The listing builds one solid part. Answer for the finished solid, in the listing's coordinates (mm). Face numbers are marked on the shaded views. Round coordinates to 2 decimals unless told otherwise and drop trailing zeros. Loops run counter-clockwise (first coordinate to the right, second up) from the corner with the lowest first, then second, coordinate; pieces in that order, holes last. Notation, with made-up numbers: M -17.75,18.25 L -7.75,18.25 A20 ccw -7.75,44.25 Z; hole C 36,59 d10. An arc over 180 degrees is marked long. Put each result on its own line as item: value. Start each with the question number.
(1) Straight lines are drawn through the part: line 1 (Z direction, x = 173.5, y = -11.25); line 2 (Z direction, x = 55.5, y = -12.5); line 3 (Z direction, x = 284.5, y = -13.75). For each, find the intervals that lie inside material, in ascending order.
(2) Section A-A, the plane x = 105 is taken. Determine the outline of the cut face in (y, z).
(3) Determine the mould class of the marked faces 1 and 2 for opening direction Z: released by +Z, released by -Z, zero draft, split by the parting line, or undercut.
(4) Section B-B, the plane z = 670 is taken. Determine the outline of the cut face in (x, y).
(5) Flat-ended cylindrical pins translate along their axes: P1, Ø8, axis at x = 130.5, z = 746.5, coming from the -Y side; P2, Ø1.5, axis at x = 344, y = -14, coming from the -Z side. Find the tip coordinate at first contact, or state that the pin passes through.
(6) Section C-C, the plane z = 704.5 is taken. Determine the outline of the cut face in (x, y), then the cut area to 3 significant figures.
```python
from build123d import *

# Parameters (mm, degrees)
F0_W      = 44.656470418
F0_H      = 33.8078811765
F1_DEPTH  = 16
F2_DEPTH  = 796
F3_DEPTH  = 196
F4_W      = 68.9578056335
F4_H      = 493.6993122101
F5_DEPTH  = 7
F6_DEPTH  = 9.7
F7_DEPTH  = 99.33
F8_DEPTH  = 99.33
F9_DEPTH  = 17.34
F10_DEPTH = 102.97
F11_W     = 35.2807044983
F11_H     = 492.0964837074
F12_DEPTH = 7
F13_DEPTH = 37.27
F14_DEPTH = 6.58
F15_DEPTH = 106.63
F16_DEPTH = 5.87
F17_DEPTH = 200
F18_DEPTH = 200
F19_DEPTH = 200
F20_DEPTH = 600
F21_DEPTH = 600
F22_DEPTH = 600
F23_R     = 3


with BuildPart() as f1:
    # F0 (on Front) → F1 (new body)
    with BuildSketch(Plane.XZ):
        with Locations((22.328235209, 16.9039405882)):
            Rectangle(F0_W, F0_H)
    extrude(amount=F1_DEPTH)

    # F2 (add): a face of the model
    f2_faces = [f1.faces().sort_by_distance(p)[0] for p in [
        (22.328235209, -8, 0),
    ]]
    extrude(f2_faces, amount=-F2_DEPTH)

    # F3 (add): a face of the model
    f3_faces = [f1.faces().sort_by_distance(p)[0] for p in [
        (0, -8, 398),
    ]]
    extrude(f3_faces, amount=-F3_DEPTH)

    # F4 (on face) → F5 (cut)
    with BuildSketch(Plane.XZ.offset(16)):
        with Locations((94.1769480705, 399.8196721077)):
            Rectangle(F4_W, F4_H)
    extrude(amount=-F5_DEPTH, mode=Mode.SUBTRACT)

    # F6 (cut): a face of the model
    f6_faces = [f1.faces().sort_by_distance(p)[0] for p in [
        (59.6980452538, -12.5, 399.8196721077),
    ]]
    extrude(f6_faces, amount=-F6_DEPTH, mode=Mode.SUBTRACT)

    # F7 (add): a face of the model
    f7_faces = [f1.faces().sort_by_distance(p)[0] for p in [
        (89.3269480705, -12.5, 646.6693282127),
    ]]
    extrude(f7_faces, amount=-F7_DEPTH)

    # F8 (cut): a face of the model
    f8_faces = [f1.faces().sort_by_distance(p)[0] for p in [
        (89.3269480705, -12.5, 646.6693282127),
    ]]
    extrude(f8_faces, amount=-F8_DEPTH, mode=Mode.SUBTRACT)

    # F9 (cut): a face of the model
    f9_faces = [f1.faces().sort_by_distance(p)[0] for p in [
        (128.6558508873, -12.5, 449.4846721077),
    ]]
    extrude(f9_faces, amount=-F9_DEPTH, mode=Mode.SUBTRACT)

    # F10 (cut): a face of the model
    f10_faces = [f1.faces().sort_by_distance(p)[0] for p in [
        (97.9969480705, -12.5, 152.9700160027),
    ]]
    extrude(f10_faces, amount=-F10_DEPTH, mode=Mode.SUBTRACT)

    # F11 (on face) → F12 (join)
    with BuildSketch(Plane.XZ.offset(9)):
        with Locations((91.7714834213, 432.6795041561)):
            Rectangle(F11_W, F11_H)
    extrude(amount=F12_DEPTH)

    # F13 (add): a face of the model
    f13_faces = [f1.faces().sort_by_distance(p)[0] for p in [
        (91.7714834213, -12.5, 678.7277460098),
    ]]
    extrude(f13_faces, amount=F13_DEPTH)

    # F14 (add): a face of the model
    f14_faces = [f1.faces().sort_by_distance(p)[0] for p in [
        (109.4118356705, -12.5, 451.3145041561),
    ]]
    extrude(f14_faces, amount=F14_DEPTH)

    # F15 (add): a face of the model
    f15_faces = [f1.faces().sort_by_distance(p)[0] for p in [
        (95.0614834213, -12.5, 186.6312623024),
    ]]
    extrude(f15_faces, amount=F15_DEPTH)

    # F16 (cut): a face of the model
    f16_faces = [f1.faces().sort_by_distance(p)[0] for p in [
        (74.1311311722, -12.5, 397.9995041561),
    ]]
    extrude(f16_faces, amount=-F16_DEPTH, mode=Mode.SUBTRACT)

    # F17 (add): a face of the model
    f17_faces = [f1.faces().sort_by_distance(p)[0] for p in [
        (196, -8, 398),
    ]]
    extrude(f17_faces, amount=F17_DEPTH)

    # F18 (cut): a face of the model
    f18_faces = [f1.faces().sort_by_distance(p)[0] for p in [
        (145.9958508873, -12.5, 397.9996721077),
    ]]
    extrude(f18_faces, amount=-F18_DEPTH, mode=Mode.SUBTRACT)

    # F19 (add): a face of the model
    f19_faces = [f1.faces().sort_by_distance(p)[0] for p in [
        (115.9918356705, -12.5, 397.9995041561),
    ]]
    extrude(f19_faces, amount=F19_DEPTH)

    # F20 (cut): a face of the model
    f20_faces = [f1.faces().sort_by_distance(p)[0] for p in [
        (197.9964834213, -12.5, 80.0012623024),
    ]]
    extrude(f20_faces, amount=-F20_DEPTH, mode=Mode.SUBTRACT)

    # F21 (add): a face of the model
    f21_faces = [f1.faces().sort_by_distance(p)[0] for p in [
        (197.9969480705, -12.5, 50.0000160027),
    ]]
    extrude(f21_faces, amount=F21_DEPTH)

    # F22 (cut): a face of the model
    f22_faces = [f1.faces().sort_by_distance(p)[0] for p in [
        (198, -8, 0),
    ]]
    extrude(f22_faces, amount=-F22_DEPTH, mode=Mode.SUBTRACT)

    # F23
    f23_edges = [f1.edges().sort_by_distance(p)[0] for p in [
        (0, -16, 698),
        (198, -16, 796),
        (396, -16, 698),
        (198, -16, 600),
        (197.996948, -16, 745.999328),
        (49.998045, -16, 697.999672),
        (345.995851, -16, 697.999672),
        (197.996948, -16, 650.000016),
        (197.996483, -16, 715.997746),
        (315.991836, -16, 697.999504),
        (197.996483, -16, 680.001262),
        (80.001131, -16, 697.999504),
    ]]
    fillet(f23_edges, radius=F23_R)


solid = f1.part
```
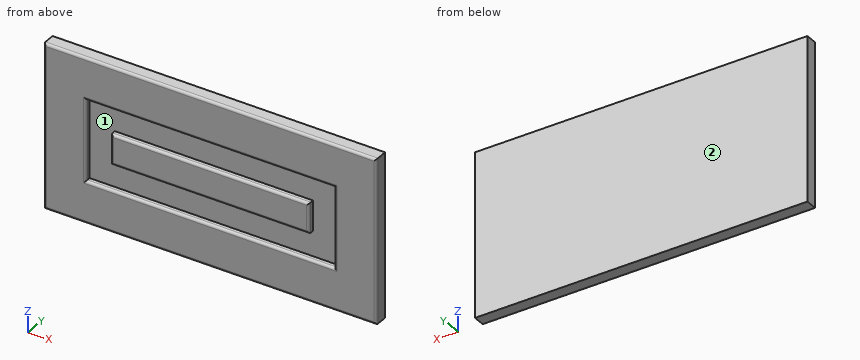
Recorded:
1. line 1: z = 600 to 650, 680 to 716, 746 to 796
1. line 2: z = 600 to 650, 746 to 796
1. line 3: z = 600.1 to 649.9, 680.1 to 715.9, 746.09 to 795.9
2. outline: M -16,603 A3 ccw -13,600 L 0,600 L 0,796 L -13,796 A3 ccw -16,793 L -16,749 A3 ccw -13,746 L -9,746 L -9,716 L -13,716 A3 ccw -16,713 L -16,683 A3 ccw -13,680 L -9,680 L -9,650 L -13,650 A3 ccw -16,647 Z
3. face 1: undercut
3. face 2: zero draft
4. outline: M 0,-13 A3 ccw 3,-16 L 47,-16 A3 ccw 50,-13 L 50,-9 L 346,-9 L 346,-13 A3 ccw 349,-16 L 393,-16 A3 ccw 396,-13 L 396,0 L 0,0 Z
5. P1: stops at y = -16
5. P2: stops at z = 600.01
6. outline: M 0,-13 A3 ccw 3,-16 L 47,-16 A3 ccw 50,-13 L 50,-9 L 80,-9 L 80,-13 A3 ccw 83,-16 L 312.99,-16 A3 ccw 315.99,-13 L 315.99,-9 L 346,-9 L 346,-13 A3 ccw 349,-16 L 393,-16 A3 ccw 396,-13 L 396,0 L 0,0 Z
6. area: 5,900 mm²
